from build123d import *

# Parameters (mm, degrees)
F0_R     = 2.1
F1_DEPTH = 1.8


with BuildPart() as f1:
    # F0 (on Top) → F1 (new body)
    with BuildSketch(Plane.XY):
        with BuildLine():
            Line((54, 68.5), (54, 28.5))
            Line((54, 28.5), (-54, 28.5))
            Line((-54, 28.5), (-54, 68.5))
            Line((-54, 68.5), (-95, 110))
            Line((-95, 110), (-105, 110))
            ThreePointArc((-105, 110), (-108.535534, 108.535534), (-110, 105))
            Line((-110, 105), (-110, 60))
            Line((-110, 60), (-101, 47.5))
            Line((-101, 47.5), (-101, -47.5))
            Line((-101, -47.5), (-110, -60))
            Line((-110, -60), (-110, -105))
            ThreePointArc((-110, -105), (-108.535534, -108.535534), (-105, -110))
            Line((-105, -110), (-95, -110))
            Line((-95, -110), (-54, -68.5))
            Line((-54, -68.5), (-54, -28.5))
            Line((-54, -28.5), (54, -28.5))
            Line((54, -28.5), (54, -68.5))
            Line((54, -68.5), (95, -110))
            Line((95, -110), (105, -110))
            ThreePointArc((105, -110), (108.535534, -108.535534), (110, -105))
            Line((110, -105), (110, -60))
            Line((110, -60), (101, -47.5))
            Line((101, -47.5), (101, 47.5))
            Line((101, 47.5), (110, 60))
            Line((110, 60), (110, 105))
            ThreePointArc((110, 105), (108.535534, 108.535534), (105, 110))
            Line((105, 110), (95, 110))
            Line((95, 110), (54, 68.5))
        make_face()
        with BuildLine():
            Line((-3.75, -21.1), (3.75, -21.1))
            ThreePointArc((3.75, -21.1), (5.25, -22.6), (3.75, -24.1))
            Line((3.75, -24.1), (-3.75, -24.1))
            ThreePointArc((-3.75, -24.1), (-5.25, -22.6), (-3.75, -21.1))
        make_face(mode=Mode.SUBTRACT)
        with Locations((58, -9)):
            Circle(F0_R, mode=Mode.SUBTRACT)
        with Locations((82, -9)):
            Circle(F0_R, mode=Mode.SUBTRACT)
        with BuildLine():
            Line((-3.75, 24.1), (3.75, 24.1))
            ThreePointArc((3.75, 24.1), (5.25, 22.6), (3.75, 21.1))
            Line((3.75, 21.1), (-3.75, 21.1))
            ThreePointArc((-3.75, 21.1), (-5.25, 22.6), (-3.75, 24.1))
        make_face(mode=Mode.SUBTRACT)
        with Locations((82, 9)):
            Circle(F0_R, mode=Mode.SUBTRACT)
    extrude(amount=F1_DEPTH)


solid = f1.part
Design review of the part built by this model. Coordinates are the model's own, in mm. A direction names the side the tool comes from. Coordinates: 2 decimals unless noted, no trailing zeros. Loops run counter-clockwise (first coordinate to the right, second up) from the corner with the lowest first, then second, coordinate; pieces in that order, holes last. Notation, with made-up numbers: (41, 56.25) - (95, 56.25) arc R11 cw to (95, 64.25) - close; hole circle Ø11 at (-16.75, 57). An arc over 180 degrees is marked (long way). Use CSV: the item, a comma, the result in double quotes. Start each with the question number.
1. Add section B-B on y = -73.5. Give the boundary of the cut face in (x, z), plus the area to 3 significant figures.
2. Add section D-D on x = -48. Give the boundary of the cut face in (y, z), plus the area to 3 significant figures.
3. For faces 5 (the flat face through (-74.213, 88.96, 0.887)), 6 (the flat face through (-105.563, 53.838, 0.887)), 7 (the flat face through (105.563, -53.838, 0.887)), list the 3-axis set-ups (+Z, -Z, +X, -X, +Y, -Y) from which the entire face can be reached by the end or side of a thin tool; tool diameter is ignored.
4. To check wall thickness, follow probe 1 along Y at (x, z) = (82, 1.2); probe 2 along X at (y, z) = (66, 1.6); probe 3 along X at (y, z) = (-101, 1.5). State the ranges of each line that lie inside material, in increasing order.
5. Clearance check with flat-ended pins moving along their axes: pin 1 (0.5 mm diameter, centred on y = -44.5, z = 1.5, fed in from -X); pin 2 (0.5 mm diameter, centred on x = -24.5, z = 0.5, fed in from -Y); pin 3 (0.9 mm diameter, centred on x = 18, z = 1, fed in from +Y). State where each tip first meets the part, or that it passes through.
6. Add section A-A on y = 36.5. Give the boundary of the cut face in (x, z), plus the area to 3 significant figures.
7. Mouldability with a two-part tool opening along X and no side actions: class faces 1 (the flat face through (105.437, 53.662, 0.887)), 2 (the flat face through (-74.787, -89.54, 0.887)), 3 (the flat face through (74.213, -88.96, 0.887)), 4 (the cylindrical face through (-108, 109, 1)) as released by +X, released by -X, zero draft, split by the parting line, or undercut.
8. Add section C-C on z = 0.9. Count the separate pieces of the cut face and the enclosed holes in it, plus the area to 3 significant figures.
Resolved:
1,outline,"(-110, 0) - (-58.94, 0) - (-58.94, 1.8) - (-110, 1.8) - close; (58.94, 0) - (110, 0) - (110, 1.8) - (58.94, 1.8) - close"
1,area,"184 mm2"
2,outline,"(-28.5, 0) - (28.5, 0) - (28.5, 1.8) - (-28.5, 1.8) - close"
2,area,"103 mm2"
3,face 5,"+Z, -Z, +Y"
3,face 6,"+Z, -Z, -X"
3,face 7,"+Z, -Z, +X"
4,probe 1,"-96.84 to -11.1, -6.9 to 6.9, 11.1 to 96.84"
4,probe 2,"-110 to -54, 54 to 110"
4,probe 3,"-110 to -86.11, 86.11 to 110"
5,pin 1,"x = -101"
5,pin 2,"y = -28.5"
5,pin 3,"y = 28.5"
6,outline,"(-101, 0) - (-54, 0) - (-54, 1.8) - (-101, 1.8) - close; (54, 0) - (101, 0) - (101, 1.8) - (54, 1.8) - close"
6,area,"169 mm2"
7,face 1,"released by +X"
7,face 2,"undercut"
7,face 3,"undercut"
7,face 4,"released by -X"
8,separate pieces,"1"
8,enclosed holes,"5"
8,area,"25,300 mm2"
